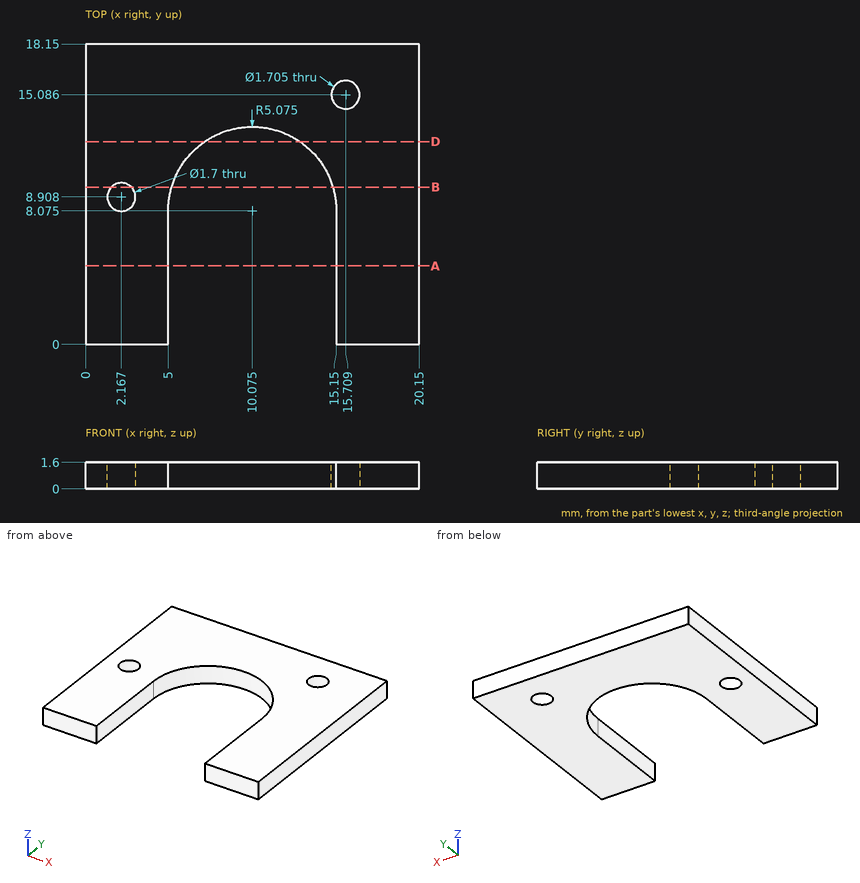
Print and shaded views of the part. All mm, measured from the part's lowest x, y and z. Coordinates: 2 decimals unless noted, no trailing zeros. Loops run counter-clockwise (first coordinate to the right, second up) from the corner with the lowest first, then second, coordinate; pieces in that order, holes last. Notation, with made-up numbers: (1.5, 41) -> (9.5, 41) arc R28 ccw to (9.5, 62) -> close; hole circle Ø7 at (-28, 78). An arc over 180 degrees is marked (long way). Use a Markdown table: item, result. Add a question column.
Item 1: Flat gauge pin, fed straight in: P1, Ø2, axis at x = 2.17, y = 8.91, coming from the -Z side. Where does the tip first touch, or does it go through?
Item 2: Probe probe 1 along X at (y, z) = (3, 0.85); probe 2 along Y at (x, z) = (2.25, 0.8); probe 3 along X at (y, z) = (11, 0.65). List the from-to ranges inside material, lowest first.
Item 3: Band-saw the part on B-B on y = 9.5. Give the number of separate pieces and of enclosed holes in the cut face, plus the area to 3 significant figures.
Item 4: Band-saw the part on D-D on y = 12.25. Write the cut outline in (x, z), plus the area to 3 significant figures.
Item 5: Band-saw the part on A-A on y = 4.75. Write the cut outline in (x, z).
Geometry says:
| question | item | result |
|---|---|---|
| 1 | P1 | z = 0 |
| 2 | probe 1 | 0 to 5, 15.15 to 20.15 |
| 2 | probe 2 | 0 to 8.06, 9.75 to 18.15 |
| 2 | probe 3 | 0 to 5.93, 14.22 to 20.15 |
| 3 | separate pieces | 3 |
| 3 | enclosed holes | 0 |
| 3 | area | 14.7 mm² |
| 4 | outline | (0, 0) -> (7.19, 0) -> (7.19, 1.6) -> (0, 1.6) -> close; (12.96, 0) -> (20.15, 0) -> (20.15, 1.6) -> (12.96, 1.6) -> close |
| 4 | area | 23.0 mm² |
| 5 | outline | (0, 0) -> (5, 0) -> (5, 1.6) -> (0, 1.6) -> close; (15.15, 0) -> (20.15, 0) -> (20.15, 1.6) -> (15.15, 1.6) -> close |
